```python
from build123d import *

# Parameters (mm, degrees)
F1_DEPTH = 1200


with BuildPart() as f1:
    # F0 (on Front) → F1 (new body)
    with BuildSketch(Plane.XZ):
        Polygon((117.767222, 265.515238), (-277.481471, 197.418033), (122.518529, 197.418033), (522.518529, 197.418033), align=None)
        Polygon((122.518529, 197.418033), (-277.481471, 197.418033), (-277.481471, -202.581967), (522.518529, -202.581967), (522.518529, 197.418033), align=None)
    extrude(amount=F1_DEPTH)


solid = f1.part
```
Geometry check sheet. Reference: the model listing, model coordinates, mm. Round coordinates to 2 decimals unless told otherwise and drop trailing zeros. Loops run counter-clockwise (first coordinate to the right, second up) from the corner with the lowest first, then second, coordinate; pieces in that order, holes last. Notation, with made-up numbers: (-33.75, 55) - (-12.75, 55) arc R6 cw to (-12.75, 61) - close; hole circle Ø7 at (-21.75, 89). An arc over 180 degrees is marked (long way). Write each question's results on one line, items separated by ' | '. Start each with the question number.
Q1. Cross-section at B-B on x = -77. Enter the section's corners in (y, z), and give its area (3 significant figures).
Q2. Gauge pin test, flat end, axial feed: P1, Ø1.5, axis at x = 146, y = -597, coming from the +Z side. Record the tip position at first contact, or that the pin passes through.
Q3. Cross-section at A-A on y = -337. Enter the section's corners in (x, z), and give its area (3 significant figures).
Q4. Cross-section at C-C on x = 40. Enter the section's corners in (y, z), and give its area (3 significant figures).
Q5. Thickness scan on line 1 (Z direction, x = 375.5, y = -842); line 2 (Z direction, x = 219.5, y = -155). Record the ranges inside material, lowest first. Write a range as [from, to].
Answers below:
1) outline: (-1200, -202.58) - (0, -202.58) - (0, 231.96) - (-1200, 231.96) - close | area: 521,000 mm²
2) P1: stops at z = 260.89
3) outline: (-277.48, -202.58) - (522.52, -202.58) - (522.52, 197.42) - (117.77, 265.52) - (-277.48, 197.42) - close | area: 347,000 mm²
4) outline: (-1200, -202.58) - (0, -202.58) - (0, 252.12) - (-1200, 252.12) - close | area: 546,000 mm²
5) line 1: z = [-202.58, 222.15] | line 2: z = [-202.58, 248.4]
